Geometry: final body of the model. Coordinates: model frame, mm. Face numbers are marked on the shaded views. A direction names the side the tool comes from. Round coordinates to 2 decimals unless told otherwise and drop trailing zeros. Order: outer loops, then holes, each group sorted by start corner. A loop starts at its lowest first (then second) coordinate and runs counter-clockwise, first axis right, second up. Notation, with made-up numbers: (35.5, 87) -> (42.5, 87) arc R23 ccw to (42.5, 107) -> close; hole circle Ø5 at (-8.75, 32.5). An arc over 180 degrees is marked (long way). Put each result on its own line as item: value.
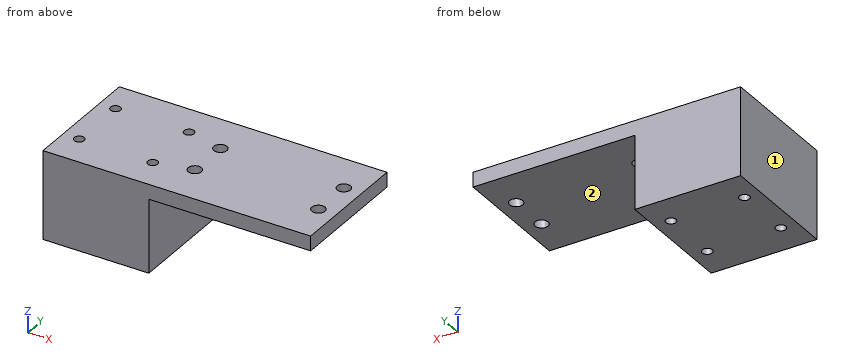
```python
from build123d import *

# Parameters (mm, degrees)
EXTRUDE_1_DEPTH    = 42
HOLE_WIZARD_M4_1_D = 4.5
HOLE_WIZARD_M3_1_D = 3.4


with BuildPart() as part:
    # 스케치1 → 보스-돌출1 (new body)
    with BuildSketch(Plane(origin=(0, 0, 0), x_dir=(1, 0, 0), z_dir=(0, 1, 0))):
        Polygon((0, 0), (0, 30), (36, 30), (36, 5), (91, 5), (91, 0), align=None)
    extrude(amount=EXTRUDE_1_DEPTH)

    # M4 여유 구멍1 (through all)
    with Locations(Plane.XY):
        with Locations((85, 28), (85, 14), (43, 28), (43, 14)):
            Hole(HOLE_WIZARD_M4_1_D / 2)

    # M3 여유 구멍1 (through all)
    with Locations(Plane.XY):
        with Locations((5.5, 31), (5.5, 11), (30.5, 31), (30.5, 11)):
            Hole(HOLE_WIZARD_M3_1_D / 2)


solid = part.part
```
1. Cut plane C-C on z = -13.25. Return loops of the section in (x, y), and give its area (3 significant figures).
Ans:
outline: (0, 0) -> (36, 0) -> (36, 42) -> (0, 42) -> close; hole circle Ø3.4 at (5.5, 11); hole circle Ø3.4 at (5.5, 31); hole circle Ø3.4 at (30.5, 11); hole circle Ø3.4 at (30.5, 31)
area: 1,480 mm²
2. Cut plane D-D on x = 43. Return loops of the section in (y, z), and give its area (3 significant figures).
Ans:
outline: (0, -5) -> (11.75, -5) -> (11.75, 0) -> (0, 0) -> close; (16.25, -5) -> (25.75, -5) -> (25.75, 0) -> (16.25, 0) -> close; (30.25, -5) -> (42, -5) -> (42, 0) -> (30.25, 0) -> close
area: 165 mm²
3. Cut plane A-A on x = 30.5. Return loops of the section in (y, z), and give its area (3 significant figures).
Ans:
outline: (0, -30) -> (9.3, -30) -> (9.3, 0) -> (0, 0) -> close; (12.7, -30) -> (29.3, -30) -> (29.3, 0) -> (12.7, 0) -> close; (32.7, -30) -> (42, -30) -> (42, 0) -> (32.7, 0) -> close
area: 1,060 mm²
4. Cut plane B-B on y = 28. Return loops of the section in (x, z), and give its area (3 significant figures).
Ans:
outline: (0, -30) -> (36, -30) -> (36, -5) -> (40.75, -5) -> (40.75, 0) -> (0, 0) -> close; (45.25, -5) -> (82.75, -5) -> (82.75, 0) -> (45.25, 0) -> close; (87.25, -5) -> (91, -5) -> (91, 0) -> (87.25, 0) -> close
area: 1,310 mm²
5. Set-up query: the marked faces 1 and 2. Return all of +Z, -Z, +X, -X, +Y, -Y with unobstructed straight access to the full face (end or side cutting, diameter ignored); none if empty.
Ans:
face 1: +Z, -Z, -X, +Y, -Y
face 2: -Z, +X, +Y, -Y
6. Material intervals for probe 1 along Y at (x, z) = (5.5, -7.5); probe 2 along Y at (x, z) = (85, -2.2); probe 3 along Z at (x, y) = (44.5, 16), sorted ascending.
Ans:
probe 1: 0 to 9.3, 12.7 to 29.3, 32.7 to 42
probe 2: 0 to 11.75, 16.25 to 25.75, 30.25 to 42
probe 3: -5 to 0
7. Contact query for flat-ended pins moving along their axis: P1, Ø1.5, axis at y = 34.5, z = -16.5, coming from the +X side; P2, Ø2, axis at x = 30.5, y = 11, coming from the +Z side; P3, Ø6, axis at x = 85, y = 14, coming from the -Z side. Output: stop coordinate, or through.
Ans:
P1: x = 36
P2: through
P3: z = -5
